Part model, mm, in its own coordinate system. Round coordinates to 2 decimals unless told otherwise and drop trailing zeros. Write each loop counter-clockwise with the first axis right and the second up, starting at its lowest first coordinate (ties: lowest second). Pieces come first, ordered by that corner, then holes.
from build123d import *

# Parameters (mm, degrees)
F0_W     = 6.35
F0_H     = 63.5
F1_DEPTH = 25.4
F2_R     = 7.62
F3_R     = 4.7625
F4_DEPTH = 25.4


with BuildPart() as f1:
    # F0 (on Front) → F1 (new body)
    with BuildSketch(Plane.XZ):
        with Locations((3.175, 31.75)):
            Rectangle(F0_W, F0_H)
    extrude(amount=F1_DEPTH)

    # F2
    f2_edges = [f1.edges().sort_by_distance(p)[0] for p in [
        (3.175, -25.4, 63.5),
        (3.175, 0, 63.5),
    ]]
    fillet(f2_edges, radius=F2_R)

    # F3 (on face) → F4 (cut)
    with BuildSketch(Plane.YZ.offset(6.35)):
        with Locations((-12.7, 52.3875)):
            Circle(F3_R)
    extrude(amount=-F4_DEPTH, mode=Mode.SUBTRACT)


solid = f1.part
Q1. Drop flat-ended pins along their axis: P1, Ø2, axis at x = 3.5, y = -19.5, coming from the +Z side; P2, Ø11, axis at y = -12.7, z = 52.39, coming from the -X side; P3, Ø3, axis at y = -12, z = 55, coming from the +X side. Give the stop position or say it passes through.
Q2. Saw through at B-B, the plane z = 49. Write the cut outline in (x, y), and give its area (3 significant figures).
Q3. Saw through at D-D, the plane y = -21.75. Write the cut outline in (x, z), and give its area (3 significant figures).
Q4. Saw through at C-C, the plane x = 3.75. Write the cut outline in (y, z) (1 decimal), and give its area (3 significant figures).
Q5. Two-plate mould, pull along Z, no slides. Class faces 1 (the flat face through (3, -13, 63.5)), 2 (the cylindrical face through (3.219, -10.502, 48.162)), 3 (the flat face through (0, -13, 31)): released by +Z, released by -Z, zero draft, split by the parting line, or undercut.
Q6. Saw through at A-A, the plane y = -12.7. Write the cut outline in (x, z) (3 decimals).
Q7. Wall check: line 1 (Z direction, x = 2.5, y = -12.7) (3 decimals); line 2 (Z direction, x = 5, y = -11); line 3 (Y direction, x = 1.5, z = 53.5). Give the ranges that are in metal, low to high.
Computed:
1. P1: stops at z = 63.47
1. P2: stops at x = 0
1. P3: passes through
2. outline: (0, -25.4) - (6.35, -25.4) - (6.35, -16.05) - (0, -16.05) - close; (0, -9.35) - (6.35, -9.35) - (6.35, 0) - (0, 0) - close
2. area: 119 mm2
3. outline: (0, 0) - (6.35, 0) - (6.35, 62.38) - (0, 62.38) - close
3. area: 396 mm2
4. outline: (-25.4, 0) - (0, 0) - (0, 55.9) arc R7.6 ccw to (-7.6, 63.5) - (-17.8, 63.5) arc R7.6 ccw to (-25.4, 55.9) - close; hole circle Ø9.5 at (-12.7, 52.4)
4. area: 1,520 mm2
5. face 1: released by +Z
5. face 2: undercut
5. face 3: zero draft
6. outline: (0, 0) - (6.35, 0) - (6.35, 47.625) - (0, 47.625) - close; (0, 57.15) - (6.35, 57.15) - (6.35, 63.5) - (0, 63.5) - close
7. line 1: z = 0 to 47.625, 57.15 to 63.5
7. line 2: z = 0 to 47.94, 56.84 to 63.5
7. line 3: y = -25.4 to -17.33, -8.07 to 0
